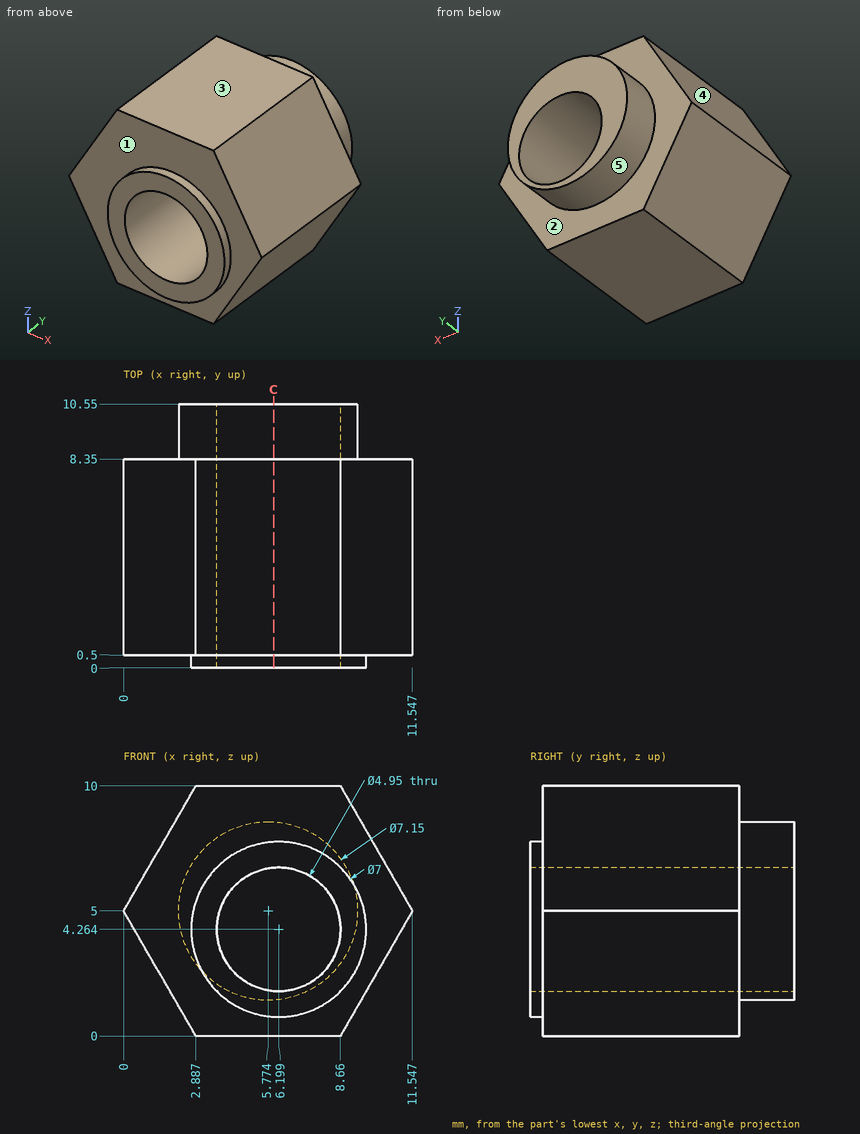
Input: dimensioned drawing with shaded views. Units: mm. Origin: part minimum x, y, z. A direction names the side the tool comes from. Coordinates: 2 decimals unless noted, no trailing zeros. Order: outer loops, then holes, each group sorted by start corner. A loop starts at its lowest first (then second) coordinate and runs counter-clockwise, first axis right, second up. Notation, with made-up numbers: M 24,81 L 68,81 A16 ccw 68,95 Z; hole C 83.5,36.25 d4. An arc over 180 degrees is marked long. Write each question's results on one line, items separated by ' | '. Start each with the question number.
Item 1: First-contact query: pin 1 Ø1.5 at (x, z) = (2.5, 1) entering from -Y; pin 2 Ø3 at (x, z) = (5.5, 3) entering from +Y; pin 3 Ø1 at (x, y) = (10, 6) entering from +Z (1 decimal); pin 4 Ø3 at (y, z) = (1.5, 7.5) entering from -X. Flat tips, straight axial feed; report the tip coordinate or a pass-through.
Item 2: Set-up query: the marked faces 4 and 5. Return all of +Z, -Z, +X, -X, +Y, -Y with unobstructed straight access to the full face (end or side cutting, diameter ignored); none if empty.
Item 3: Draft query along Y for the marked faces 1, 2 and 3. Return one class per face: pulls with the +Y half, pulls with the -Y half, needs draft (parallel to the pull), parting line crosses it, or undercut.
Item 4: Cut plane C-C (x = 6). Return loops of the section in (y, z).
Item 5: Line query: probe 1 along Y at (x, z) = (9, 2); probe 2 along X at (y, z) = (4, 2.5) (1 decimal); probe 3 along X at (y, z) = (6.5, 3) (1 decimal). Output: solid intervals per line, ascending.
Checked values:
1) pin 1: stops at y = 0.5 | pin 2: stops at y = 10.55 | pin 3: stops at z = 8.5 | pin 4: stops at x = 0.58
2) face 4: +Z, -X, +Y, -Y | face 5: +Y
3) face 1: pulls with the -Y half | face 2: pulls with the +Y half | face 3: needs draft
4) outline: M 0,0.77 L 0.5,0.77 L 0.5,0 L 8.35,0 L 8.35,1.43 L 10.55,1.43 L 10.55,1.8 L 0,1.8 Z; M 0,6.73 L 10.55,6.73 L 10.55,8.57 L 8.35,8.57 L 8.35,10 L 0.5,10 L 0.5,7.76 L 0,7.76 Z
5) probe 1: y = 0.5 to 8.35 | probe 2: x = 1.4 to 4.5, 7.9 to 10.1 | probe 3: x = 1.2 to 4.1, 8.3 to 10.4
